Could you check a few things on this model? Use its own coordinates, in mm. A direction names the side the tool comes from. Coordinates: 2 decimals unless noted, no trailing zeros. Write each loop counter-clockwise with the first axis right and the second up, starting at its lowest first coordinate (ties: lowest second). Pieces come first, ordered by that corner, then holes.
Item 1: I want a section at A-A on z = 22. State how many separate pieces and enclosed holes the cut face has, then the cut area to 3 significant figures.
Item 2: I want a section at D-D on x = -2. Please give me the cut outline in (y, z).
Item 3: Thinking about a two-plate mould opening in Y: for faces 1 (the flat face through (2, 0, 40)), 2 (the cylindrical face through (1.036, -4.93, 20.689)), 3 (the flat face through (2, 3, 56.465)), 4 (the cylindrical face through (-4.514, 21.993, 28.014)), which applies, +Y half, -Y half, draft (parallel to the pull), parting line (faces both ways), or undercut?
Item 4: I want a section at C-C on z = 47. Please give me the cut outline in (x, y), then the cut area to 3 significant figures.
Item 5: I want a section at B-B on y = -5. Please give me the cut outline in (x, z), then the cut area to 3 significant figures.
Item 6: For P1, Ø6, axis at x = 1, z = 22.5, coming from the +Y side; P2, Ø8, axis at x = 6.5, z = 27.5, coming from the -Y side; P3, Ø8, axis at x = 9.5, z = 37.5, coming from the +Y side; P4, Ø5, axis at x = -2.5, z = 48.5, coming from the +Y side, each with a flat end and sliding along its axis, tell me the tip position at first contact or that it passes through.
Item 7: Which directions (+Z, -Z, +X, -X, +Y, -Y) give clear straight access to the entire face, cutting with the end or side of a thin tool? Please do faces 5 (the flat face through (2, 5, 49)), 6 (the flat face through (2, -3, 23.154)), 7 (the flat face through (-7.366, 5, 29)).
Item 8: If I drill on probe 1 along Z at (x, y) = (11.5, -0.5); probe 2 along Z at (x, y) = (7.25, 9.5); probe 3 along Y at (x, z) = (-1.5, 44.5), over which ranges is the centre line in solid material (lowest first)?
from build123d import *

# Parameters (mm, degrees)
SKETCH_1_W          = 20
SKETCH_1_H          = 40
EXTRUDE_1_DEPTH     = 5
SKETCH_2_W          = 20
SKETCH_2_H          = 20
EXTRUDE_2_DEPTH     = 20
SKETCH_3_R          = 4.15
CUT_EXTRUDE_1_DEPTH = 42.044142746
FILLET_1_R          = 10
SKETCH_6_W          = 20
SKETCH_6_H          = 25.791536141
CUT_EXTRUDE_3_DEPTH = 54.65112416
SKETCH_7_W          = 20
SKETCH_7_H          = 5
EXTRUDE_5_DEPTH     = 10
SKETCH_8_W          = 20
SKETCH_8_H          = 5
EXTRUDE_6_DEPTH     = 10
SKETCH_10_R         = 1.6
CUT_EXTRUDE_5_DEPTH = 45.828803841
SKETCH_11_W         = 20
SKETCH_11_H         = 5
EXTRUDE_7_DEPTH     = 20
SKETCH_12_R         = 2.6
CUT_EXTRUDE_7_DEPTH = 82.655934826
SKETCH_13_W         = 20
SKETCH_13_H         = 21.689007925
CUT_EXTRUDE_8_DEPTH = 82.655934826


with BuildPart() as part:
    # 草图1 → 凸台-拉伸1 (new body)
    with BuildSketch(Plane(origin=(0, 0, 0), x_dir=(1, 0, 0), z_dir=(0, 1, 0))):
        with Locations((2.634146341, -28.154142811)):
            Rectangle(SKETCH_1_W, SKETCH_1_H)
    extrude(amount=EXTRUDE_1_DEPTH)

    # 草图2 → 凸台-拉伸2 (add)
    with BuildSketch(Plane(origin=(0, 5, 0), x_dir=(1, 0, 0), z_dir=(0, 1, 0))):
        with Locations((2.634146341, -28.154142811)):
            Rectangle(SKETCH_2_W, SKETCH_2_H)
    extrude(amount=EXTRUDE_2_DEPTH)

    # 草图3 → 切除-拉伸1 (cut, through all)
    with BuildSketch(Plane.XY.offset(38.154142811)):
        with Locations((2.634146341, 15)):
            Circle(SKETCH_3_R)
    extrude(amount=-CUT_EXTRUDE_1_DEPTH, mode=Mode.SUBTRACT)

    # 圆角1
    fillet_1_edges = [part.edges().sort_by_distance(p)[0] for p in [
        (12.634146341, 25, 28.154142811),
        (-7.365853659, 25, 28.154142811),
    ]]
    fillet(fillet_1_edges, radius=FILLET_1_R - 0.0001)  # a hair under: the kernel refuses the full size

    # 草图6 → 切除-拉伸3 (cut, through all)
    with BuildSketch(Plane(origin=(0, 5, 0), x_dir=(1, 0, 0), z_dir=(0, 1, 0))):
        with Locations((2.634146341, -5.25837474)):
            Rectangle(SKETCH_6_W, SKETCH_6_H)
    extrude(amount=-CUT_EXTRUDE_3_DEPTH, mode=Mode.SUBTRACT)

    # 草图7 → 凸台-拉伸5 (add)
    with BuildSketch(Plane.XZ):
        with Locations((2.634146341, 20.654142811)):
            Rectangle(SKETCH_7_W, SKETCH_7_H)
    extrude(amount=EXTRUDE_5_DEPTH)

    # 草图8 → 凸台-拉伸6 (add)
    with BuildSketch(Plane.XY.offset(48.154142811)):
        with Locations((2.634146341, 2.5)):
            Rectangle(SKETCH_8_W, SKETCH_8_H)
    extrude(amount=EXTRUDE_6_DEPTH)

    # 草图10 → 切除-拉伸5 (cut, through all)
    with BuildSketch(Plane.XY.offset(23.154142811)):
        with Locations((2.634146341, -5)):
            Circle(SKETCH_10_R)
    extrude(amount=-CUT_EXTRUDE_5_DEPTH, mode=Mode.SUBTRACT)

    # 草图11 → 凸台-拉伸7 (add)
    with BuildSketch(Plane.XY.offset(58.154142811)):
        with Locations((2.634146341, 2.5)):
            Rectangle(SKETCH_11_W, SKETCH_11_H)
    extrude(amount=EXTRUDE_7_DEPTH)

    # 草图12 → 切除-拉伸7 (cut, through all)
    with BuildSketch(Plane(origin=(0, 5, 0), x_dir=(1, 0, 0), z_dir=(0, 1, 0))):
        with Locations(Location((2.634146341, -46.221727325, 0), (0, 0, 270))):
            Circle(SKETCH_12_R)
        with Locations(Location((2.634146341, -72.110167443, 0), (0, 0, 270))):
            Circle(SKETCH_12_R)
    extrude(amount=-CUT_EXTRUDE_7_DEPTH, mode=Mode.SUBTRACT)

    # 草图13 → 切除-拉伸8 (cut, through all)
    with BuildSketch(Plane(origin=(0, 5, 0), x_dir=(1, 0, 0), z_dir=(0, 1, 0))):
        with Locations((2.634146341, -67.309638849)):
            Rectangle(SKETCH_13_W, SKETCH_13_H)
    extrude(amount=-CUT_EXTRUDE_8_DEPTH, mode=Mode.SUBTRACT)


solid = part.part
Response values:
1. separate pieces: 1
1. enclosed holes: 2
1. area: 595 mm2
2. outline: (-10, 18.15) - (23.86, 18.15) - (23.86, 38.15) - (5, 38.15) - (5, 56.47) - (0, 56.47) - (0, 23.15) - (-10, 23.15) - close
3. face 1: -Y half
3. face 2: undercut
3. face 3: draft
3. face 4: +Y half
4. outline: (-7.37, 0) - (0.15, 0) - (0.15, 5) - (-7.37, 5) - close; (5.11, 0) - (12.63, 0) - (12.63, 5) - (5.11, 5) - close
4. area: 75.2 mm2
5. outline: (-7.37, 18.15) - (1.03, 18.15) - (1.03, 23.15) - (-7.37, 23.15) - close; (4.23, 18.15) - (12.63, 18.15) - (12.63, 23.15) - (4.23, 23.15) - close
5. area: 84.0 mm2
6. P1: stops at y = 25
6. P2: stops at y = 0
6. P3: stops at y = 24.58
6. P4: stops at y = 5
7. face 5: +Z, +X, -X, +Y
7. face 6: +Z, +X, -X, -Y
7. face 7: +Z, -Z, -X, +Y, -Y
8. probe 1: z = 18.15 to 23.15
8. probe 2: z = 18.15 to 38.15
8. probe 3: y = 0 to 5
